Here's how the part is built. I have some questions about the finished solid (model axes, mm). A direction names the side the tool comes from. Coordinates: 2 decimals unless noted, no trailing zeros. Order: outer loops, then holes, each group sorted by start corner. A loop starts at its lowest first (then second) coordinate and runs counter-clockwise, first axis right, second up. Notation, with made-up numbers: M 42.5,36 L 69.5,36 A38 ccw 69.5,75 Z; hole C 74,16.5 d5. An arc over 180 degrees is marked long. Answer as CSV lines item,"result". Start each with the question number.
```python
from build123d import *

# Parameters (mm, degrees)
F1_DEPTH = 1
F3_DEPTH = 2
F5_DEPTH = 4
F7_DEPTH = 25


with BuildPart() as f1:
    # F0 (on Front) → F1 (new body)
    with BuildSketch(Plane.XZ):
        with BuildLine():
            Line((7, -33), (7, 0))
            Line((7, 0), (-7, 0))
            Line((-7, 0), (-7, -37))
            Line((-7, -37), (14.751387, -47.142838))
            Line((14.751387, -47.142838), (12.215677, -52.580685))
            Line((12.215677, -52.580685), (34.210687, -59.305234))
            ThreePointArc((34.210687, -59.305234), (35.730719, -58.472537), (35.343644, -56.783142))
            Line((35.343644, -56.783142), (7, -33))
        make_face()
    extrude(amount=F1_DEPTH)

    # F2 (on face) → F3 (join)
    with BuildSketch(Plane(origin=(0, 0, 0), x_dir=(-1, 0, 0), z_dir=(0, 1, 0))):
        Polygon((7, -37), (7, 0), (6, 0), (6, -37.466308), align=None)
    extrude(amount=F3_DEPTH)

    # F4 (on face) → F5 (join)
    with BuildSketch(Plane(origin=(0, 0, 0), x_dir=(-1, 0, 0), z_dir=(0, 1, 0))):
        Polygon((-34.700857, -57.549186), (-6, -33.466308), (-6, 0), (-7, 0), (-7, -33), (-35.343644, -56.783142), align=None)
        Polygon((-12.215677, -52.580685), (-12.642449, -51.66547), (-34.503058, -58.348929), (-34.210687, -59.305234), align=None)
    extrude(amount=F5_DEPTH)

    # F6 (on face) → F7 (cut)
    with BuildSketch(Plane.XZ.offset(1)):
        with BuildLine():
            ThreePointArc((2.5, -9.5), (0, -7), (-2.5, -9.5))
            Line((-2.5, -9.5), (-2.5, -33.5))
            ThreePointArc((-2.5, -33.5), (0, -36), (2.5, -33.5))
            Line((2.5, -33.5), (2.5, -9.5))
        make_face()
    extrude(amount=-F7_DEPTH, mode=Mode.SUBTRACT)


solid = f1.part
```
1) If we mould it in two halves opening along Z, with no side actions, what happens to faces 4 (the face through (35.72, -0.49, -58.5)), 5 (the face through (23.42, 1.97, -54.96)), 6 (the face through (20.973, 1.465, -44.725)), 7 (the face through (5.5, 0, -29.5))? For each: released by +Z, released by -Z, zero draft, split by the parting line, or undercut.
2) Suppose I cut it at C-C on x = 14. Please give me the cut outline in (y, z), plus the area to 3 significant figures.
3) I need wall thicknesses on line 1 (X direction, y = 0.75, z = -26); line 2 (X direction, y = -0.1, z = -14.5); line 3 (X direction, y = 2.65, z = -27.5). Which ranges of each line are inside material? Lowest first, please. Write a range as [from, to].
4) Which directions (+Z, -Z, +X, -X, +Y, -Y) give clear straight access to the entire face, cutting with the end or side of a thin tool? Please do faces 1 (the face through (20.551, 1.972, -45.676)), 2 (the face through (7, 1, -16)), 3 (the face through (0.1, -0.5, -7)).
5) Suppose I cut it at D-D on x = 26. Please give me the cut outline in (y, z), plus the area to 3 significant figures.
6) Will these pins go through, and if not, where does the flat tip stop? pin 1 Ø1 at (y, z) = (0.5, -18) entering from +X; pin 2 Ø1.1 at (x, z) = (-6.5, -16) entering from +Y; pin 3 Ø10 at (x, z) = (15, -13.5) entering from +Y.
7) Suppose I cut it at A-A on y = 2.8. Please give me the cut outline in (x, z), plus the area to 3 significant figures.
8) Suppose I cut it at B-B on z = -12.5. Please give me the cut outline in (x, y), plus the area to 3 significant figures.
Output:
1,face 4,"split by the parting line"
1,face 5,"undercut"
1,face 6,"released by +Z"
1,face 7,"undercut"
2,outline,"M -1,-53.13 L 4,-53.13 L 4,-52.08 L 0,-52.08 L 0,-48.75 L -1,-48.75 Z; M -1,-46.79 L 0,-46.79 L 0,-40.18 L 4,-40.18 L 4,-38.87 L -1,-38.87 Z"
2,area,"21.7 mm²"
3,line 1,"[-7, -6], [6, 7]"
3,line 2,"[-7, -2.5], [2.5, 7]"
3,line 3,"[6, 7]"
4,face 1,"+Y"
4,face 2,"+Z, +X, +Y, -Y"
4,face 3,"+Y, -Y"
5,outline,"M -1,-56.79 L 4,-56.79 L 4,-55.75 L 0,-55.75 L 0,-50.25 L 4,-50.25 L 4,-48.94 L -1,-48.94 Z"
5,area,"17.3 mm²"
6,pin 1,"x = 7"
6,pin 2,"y = 2"
6,pin 3,"through"
7,outline,"M 6,-33.47 L 34.7,-57.55 L 35.34,-56.78 L 7,-33 L 7,0 L 6,0 Z; M 12.22,-52.58 L 34.21,-59.31 L 34.5,-58.35 L 12.64,-51.67 Z"
7,area,"93.4 mm²"
8,outline,"M -7,-1 L -2.5,-1 L -2.5,0 L -6,0 L -6,2 L -7,2 Z; M 2.5,-1 L 7,-1 L 7,4 L 6,4 L 6,0 L 2.5,0 Z"
8,area,"15.0 mm²"
